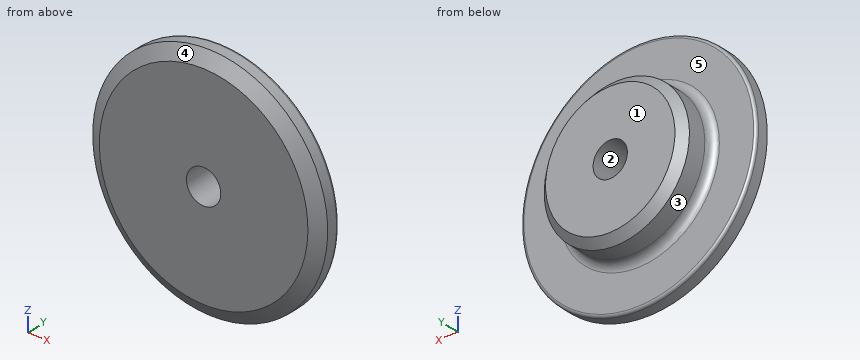
from build123d import *

# Parameters (mm, degrees)
F0_W     = 13
F0_H     = 21
F0_W_2   = 8
F0_H_2   = 17
F2_R     = 3
F3_R     = 1
F4_SIZE  = 3
F5_SIZE2 = 3
F5_SIZE  = 5


with BuildPart() as f1:
    # F0 (on Right) → F1 (revolve)
    with BuildSketch(Plane.YZ):
        with Locations((14.5, 17)):
            Rectangle(F0_W, F0_H)
        with Locations((4, 17)):
            Rectangle(F0_W_2, F0_H)
        with Locations((4, 36)):
            Rectangle(F0_W_2, F0_H_2)
    revolve(axis=Axis((0, 10.5, 0), (0, 1, 0)))

    # F2
    f2_edges = [f1.edges().sort_by_distance(p)[0] for p in [
        (0, 8, -27.5),
    ]]
    fillet(f2_edges, radius=F2_R)

    # F3
    f3_edges = [f1.edges().sort_by_distance(p)[0] for p in [
        (0, 8, -44.5),
    ]]
    fillet(f3_edges, radius=F3_R)

    # F4
    f4_edges = [f1.edges().sort_by_distance(p)[0] for p in [
        (0, 21, -27.5),
    ]]
    chamfer(f4_edges, length=F4_SIZE)

    # F5
    f5_edges = [f1.edges().sort_by_distance(p)[0] for p in [
        (0, 0, -44.5),
    ]]
    chamfer(f5_edges, length=F5_SIZE, length2=F5_SIZE2)


solid = f1.part
Read the model definition and answer for the solid it produces. Units are mm, in the model's axes. Face numbers are marked on the shaded views. A direction names the side the tool comes from. Give positions to 0.01 mm unless a question says otherwise; leave off trailing zeros. Loops run counter-clockwise (first coordinate to the right, second up) from the corner with the lowest first, then second, coordinate; pieces in that order, holes last. Notation, with made-up numbers: (15, 30.25) -> (72, 30.25) arc R14 ccw to (72, 39.25) -> close; hole circle Ø4 at (65, 26). An arc over 180 degrees is marked (long way). Use a Markdown table: item, result.
Q1. Each of these flat-tipped pins is pushed along its axis until it touches: pin 1 (3 mm diameter, centred on x = -4, y = 4, fed in from +Z); pin 2 (8 mm diameter, centred on x = -23.5, y = 17, fed in from +Z); pin 3 (3 mm diameter, centred on y = 2, z = 4, fed in from +X). Where does it stop, or does it pass through?
Solved:
| item | result |
|---|---|
| pin 1 | stops at z = 44.43 |
| pin 2 | stops at z = 19.39 |
| pin 3 | stops at x = 44.41 |
Q2. Determine the mould class of the marked faces 1, 2 and 3 for opening direction Z: pulls with the +Z half, pulls with the -Z half, needs draft (parallel to the pull), parting line crosses it, or undercut.
Solved:
| item | result |
|---|---|
| face 1 | needs draft |
| face 2 | undercut |
| face 3 | parting line crosses it |
Q3. Section C-C, the plane y = 14.5 is taken. Determine the outline of the cut face in (x, z).
Solved:
| item | result |
|---|---|
| outline | circle Ø55 at (0, 0); hole circle Ø13 at (0, 0) |
Q4. Find the intervals of material crossed by line 1 along X through (y, z) = (5, 0); line 2 along X through (y, z) = (13.25, 0); line 3 along Y through (x, z) = (-20, -29), in increasing order.
Solved:
| item | result |
|---|---|
| line 1 | x = -44.5 to -6.5, 6.5 to 44.5 |
| line 2 | x = -27.5 to -6.5, 6.5 to 27.5 |
| line 3 | y = 0 to 8 |
Q5. Section B-B, the plane z = 0 is taken. Determine the outline of the cut face in (x, y).
Solved:
| item | result |
|---|---|
| outline | (-44.5, 3) -> (-39.5, 0) -> (-6.5, 0) -> (-6.5, 21) -> (-24.5, 21) -> (-27.5, 18) -> (-27.5, 11) arc R3 cw to (-30.5, 8) -> (-43.5, 8) arc R1 ccw to (-44.5, 7) -> close; (6.5, 0) -> (39.5, 0) -> (44.5, 3) -> (44.5, 7) arc R1 ccw to (43.5, 8) -> (30.5, 8) arc R3 cw to (27.5, 11) -> (27.5, 18) -> (24.5, 21) -> (6.5, 21) -> close |
Q6. A tool of negligible diameter and unlimited length cuts with its end or side. For the marked faces 4 and 5, from which of +Z, -Z, +X, -X, +Y, -Y can it reach the whole face along a straight path? Write none if from no direction.
Solved:
| item | result |
|---|---|
| face 4 | -Y |
| face 5 | +Y |
Q7. Section A-A, the plane x = 0 is taken. Determine the outline of the cut face in (y, z).
Solved:
| item | result |
|---|---|
| outline | (0, -39.5) -> (3, -44.5) -> (7, -44.5) arc R1 ccw to (8, -43.5) -> (8, -30.5) arc R3 cw to (11, -27.5) -> (18, -27.5) -> (21, -24.5) -> (21, -6.5) -> (0, -6.5) -> close; (0, 6.5) -> (21, 6.5) -> (21, 24.5) -> (18, 27.5) -> (11, 27.5) arc R3 cw to (8, 30.5) -> (8, 43.5) arc R1 ccw to (7, 44.5) -> (3, 44.5) -> (0, 39.5) -> close |
Q8. Section D-D, the plane y = 4.25 is taken. Determine the outline of the cut face in (x, z), then the cut area to 3 significant figures.
Solved:
| item | result |
|---|---|
| outline | circle Ø89 at (0, 0); hole circle Ø13 at (0, 0) |
| area | 6,090 mm^2 |
